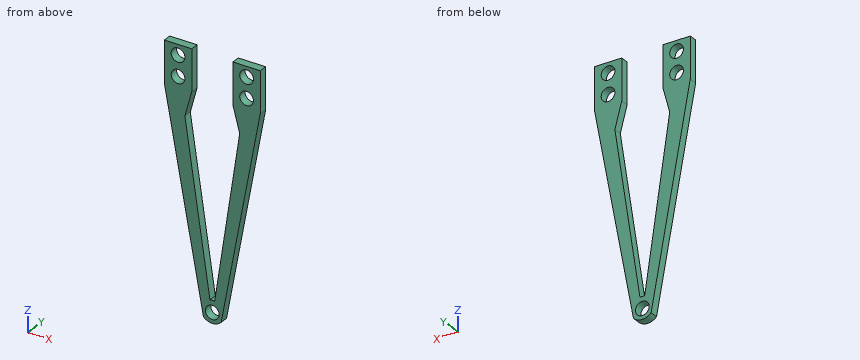
```python
from build123d import *

# Parameters (mm, degrees)
SKETCH1_R           = 5
BOSS_EXTRUDE1_DEPTH = 6
CUT_EXTRUDE1_DEPTH  = 10


with BuildPart() as part:
    # Sketch1 → Boss-Extrude1 (new body)
    with BuildSketch(Plane(origin=(0, 0, 0), x_dir=(1, 0, 0), z_dir=(0, 1, 0))):
        with BuildLine():
            Line((-35, -15), (35, -15))
            Line((35, -15), (35, 15))
            Line((35, 15), (6.447368421, 170))
            ThreePointArc((6.447368421, 170), (0, 172.670587442), (-6.447368421, 170))
            Line((-6.447368421, 170), (-35, 15))
            Line((-35, 15), (-35, -15))
        make_face()
        with Locations(Location((0, 165, 0), (0, 0, 270))):
            Circle(SKETCH1_R, mode=Mode.SUBTRACT)
        with Locations(Location((-25, 7.5, 0), (0, 0, 270))):
            Circle(SKETCH1_R, mode=Mode.SUBTRACT)
        with Locations(Location((-25, -7.5, 0), (0, 0, 270))):
            Circle(SKETCH1_R, mode=Mode.SUBTRACT)
        with Locations(Location((25, 7.5, 0), (0, 0, 90))):
            Circle(SKETCH1_R, mode=Mode.SUBTRACT)
        with Locations(Location((25, -7.5, 0), (0, 0, 90))):
            Circle(SKETCH1_R, mode=Mode.SUBTRACT)
    extrude(amount=BOSS_EXTRUDE1_DEPTH)

    # Sketch6 → Cut-Extrude1 (cut)
    with BuildSketch(Plane(origin=(0, 6, 0), x_dir=(1, 0, 0), z_dir=(0, 1, 0))):
        with BuildLine():
            Line((-15, -15), (-15, 15))
            Line((-15, 15), (-20, 33.595074374))
            Line((-20, 33.595074374), (-1.721816463, 156.693521977))
            ThreePointArc((-1.721816463, 156.693521977), (0, 156.566387575), (1.721816463, 156.693521977))
            Line((1.721816463, 156.693521977), (20, 33.595074374))
            Line((20, 33.595074374), (15, 15))
            Line((15, 15), (15, -15))
            Line((15, -15), (-15, -15))
        make_face()
    extrude(amount=-CUT_EXTRUDE1_DEPTH, mode=Mode.SUBTRACT)


solid = part.part
```
The listing builds one solid part. Answer for the finished solid, in the listing's coordinates (mm). Coordinates: 2 decimals unless noted, no trailing zeros. Write each loop counter-clockwise with the first axis right and the second up, starting at its lowest first coordinate (ties: lowest second). Pieces come first, ordered by that corner, then holes. Notation, with made-up numbers: (-16, 61) - (16, 61) arc R31 ccw to (16, 94) - close; hole circle Ø9 at (1.5, 46.5). An arc over 180 degrees is marked (long way). One line per item, written item: value.
1) Consider line 1 along X through (y, z) = (3.75, 7.5); line 2 along X through (y, z) = (3.75, -77); line 3 along X through (y, z) = (1.5, -119). Determine where each line is inside the solid, lowest interval first. Write a range as from..to.
Geometry check:
line 1: x = -35..-30, -20..-15, 15..20, 30..35
line 2: x = -23.58..-13.56, 13.56..23.58
line 3: x = -15.84..-7.32, 7.32..15.84
2) Find section C-C (y = 5). Give the vertices of the cut face in (x, z), and give its area (3 significant figures).
Geometry check:
outline: (-35, -15) - (-6.45, -170) arc R9.12 ccw to (6.45, -170) - (35, -15) - (35, 15) - (15, 15) - (15, -15) - (20, -33.6) - (1.72, -156.69) arc R11.72 ccw to (-1.72, -156.69) - (-20, -33.6) - (-15, -15) - (-15, 15) - (-35, 15) - close; hole circle Ø10 at (-25, -7.5); hole circle Ø10 at (-25, 7.5); hole circle Ø10 at (0, -165); hole circle Ø10 at (25, -7.5); hole circle Ø10 at (25, 7.5)
area: 3,930 mm2
3) Each of these flat-tipped pins is pushed along its axis until it touches: pin 1 Ø1.5 at (y, z) = (4, -117.5) entering from +X; pin 2 Ø9 at (x, z) = (-25, 7.5) entering from -Y. Where does it stop, or does it pass through?
Geometry check:
pin 1: stops at x = 16.26
pin 2: passes through
4) Find section B-B (x = 0). Give the vertices of the cut face in (y, z).
Geometry check:
outline: (0, -172.67) - (6, -172.67) - (6, -170) - (0, -170) - close; (0, -160) - (6, -160) - (6, -156.57) - (0, -156.57) - close
5) Find section D-D (z = -146). Give the vertices of the cut face in (x, y).
Geometry check:
outline: (-10.87, 0) - (-3.31, 0) - (-3.31, 6) - (-10.87, 6) - close; (3.31, 0) - (10.87, 0) - (10.87, 6) - (3.31, 6) - close
6) Find section A-A (z = -7.5). Give the vertices of the cut face in (x, y), and give its area (3 significant figures).
Geometry check:
outline: (-35, 0) - (-30, 0) - (-30, 6) - (-35, 6) - close; (-20, 0) - (-15, 0) - (-15, 6) - (-20, 6) - close; (15, 0) - (20, 0) - (20, 6) - (15, 6) - close; (30, 0) - (35, 0) - (35, 6) - (30, 6) - close
area: 120 mm2
